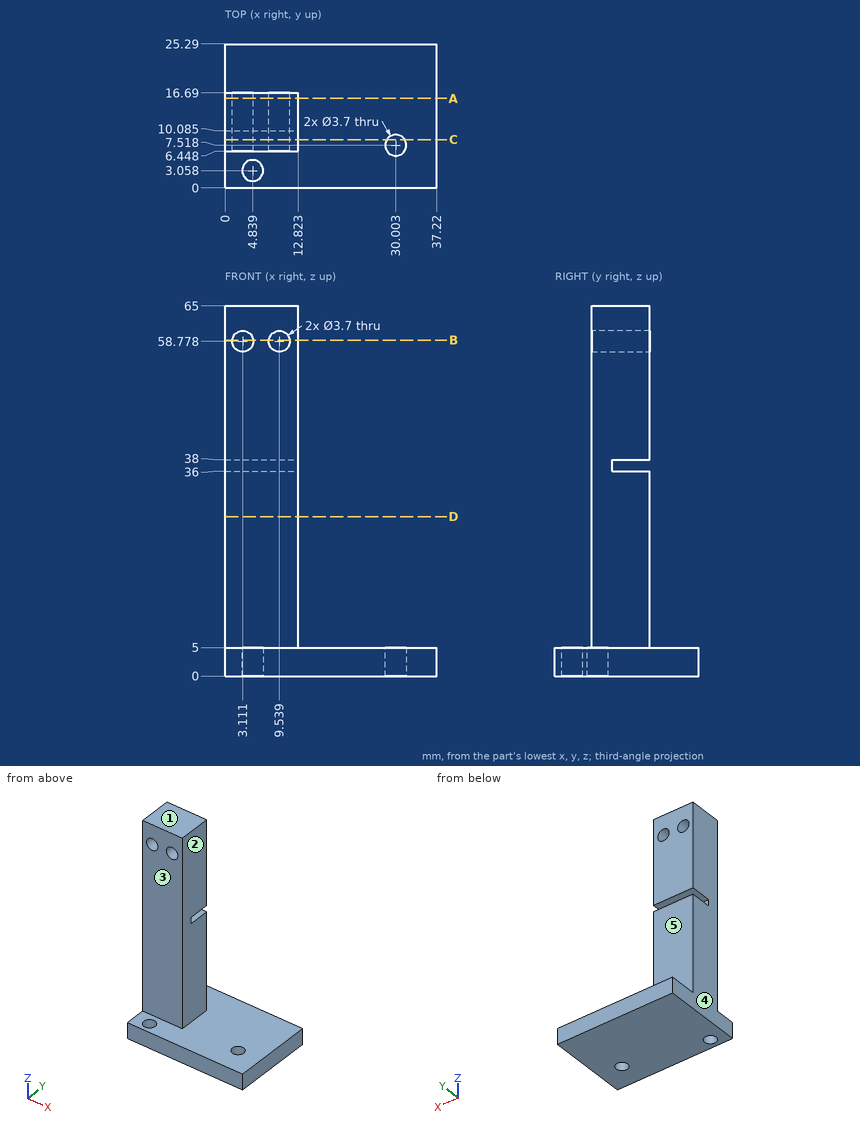
Geometry check sheet. Reference: drawing and pictorial views, mm from the part's lowest x, y, z. A direction names the side the tool comes from. Give positions to 0.01 mm unless a question says otherwise; leave off trailing zeros. Loops run counter-clockwise (first coordinate to the right, second up) from the corner with the lowest first, then second, coordinate; pieces in that order, holes last. Notation, with made-up numbers: (-26.75, 69) -> (3.25, 69) arc R29 ccw to (3.25, 100) -> close; hole circle Ø6 at (31, 45.25). An arc over 180 degrees is marked (long way). Answer in a Markdown table with one row per item. Add a question column.
1) Cross-section at B-B on z = 59. Record the boundary of the cut face in (x, y) (1 decimal).
2) Cross-section at D-D on z = 28. Record the boundary of the cut face in (x, y), and give its area (3 significant figures).
3) Material ranges on probe 1 along X at (y, z) = (15.5, 12); probe 2 along Y at (x, z) = (5, 57.5); probe 3 along Z at (x, y) = (13.5, 19.5), recorded low to high. Write a range as from..to.
4) Set-up check for the marked faces 1, 2, 3, 4 and 5: record each of +Z, -Z, +X, -X, +Y, -Y from which the full face is reachable in a straight line by a thin tool's end or side.
5) Cross-section at A-A on y = 15.75. Record the boundary of the cut face in (x, z).
6) Gauge pin test, flat ends, axial feed: P1, Ø6.5, axis at x = 4, z = 35.5, coming from the -Y side; P2, Ø8, axis at y = 16.5, z = 54.5, coming from the +X side; P3, Ø6.5, axis at x = 6.5, z = 47.5, coming from the +Y side. Record the tip position at first contact, or that the pin passes through.
7) Cross-section at C-C on y = 8.5. State how many separate pieces and enclosed holes the cut face has.
Outcome:
| question | item | result |
|---|---|---|
| 1 | outline | (0, 6.4) -> (1.3, 6.4) -> (1.3, 16.7) -> (0, 16.7) -> close; (4.9, 6.4) -> (7.7, 6.4) -> (7.7, 16.7) -> (4.9, 16.7) -> close; (11.4, 6.4) -> (12.8, 6.4) -> (12.8, 16.7) -> (11.4, 16.7) -> close |
| 2 | outline | (0, 6.45) -> (12.82, 6.45) -> (12.82, 16.69) -> (0, 16.69) -> close |
| 2 | area | 131 mm^2 |
| 3 | probe 1 | x = 0..12.82 |
| 3 | probe 2 | y = 6.45..16.69 |
| 3 | probe 3 | z = 0..5 |
| 4 | face 1 | +Z, +X, -X, +Y, -Y |
| 4 | face 2 | +Z, +X, +Y, -Y |
| 4 | face 3 | +Z, +X, -X, -Y |
| 4 | face 4 | +Z, -Z, -X, +Y, -Y |
| 4 | face 5 | +Z, +X, -X, +Y |
| 5 | outline | (0, 0) -> (37.22, 0) -> (37.22, 5) -> (12.82, 5) -> (12.82, 36) -> (0, 36) -> close; (0, 38) -> (12.82, 38) -> (12.82, 65) -> (0, 65) -> close; hole circle Ø3.7 at (3.11, 58.78); hole circle Ø3.7 at (9.54, 58.78) |
| 6 | P1 | stops at y = 6.45 |
| 6 | P2 | stops at x = 12.82 |
| 6 | P3 | stops at y = 16.69 |
| 7 | separate pieces | 2 |
| 7 | enclosed holes | 2 |
